Design review of the part built by this model. Coordinates are the model's own, in mm. Round coordinates to 2 decimals unless told otherwise and drop trailing zeros. Loops run counter-clockwise (first coordinate to the right, second up) from the corner with the lowest first, then second, coordinate; pieces in that order, holes last. Notation, with made-up numbers: M -20,-14 L 2,-14 A5 ccw 2,-7 Z; hole C 27.25,50.25 d3. An arc over 180 degrees is marked long. Answer as CSV lines item,"result". Start each with the question number.
from build123d import *

# Parameters (mm, degrees)
F0_R     = 24.5
F0_R_2   = 1.75
F0_R_3   = 1
F0_W     = 10
F0_H     = 24
F1_DEPTH = 6.35


with BuildPart() as f1:
    # F0 (on Top) → F1 (new body)
    with BuildSketch(Plane.XY):
        Circle(F0_R)
        with Locations((0, -18.5)):
            Circle(F0_R_2, mode=Mode.SUBTRACT)
        with Locations((-18.5, 0)):
            Circle(F0_R_2, mode=Mode.SUBTRACT)
        with Locations((-9, -9)):
            Circle(F0_R_3, mode=Mode.SUBTRACT)
        Rectangle(F0_W, F0_H, mode=Mode.SUBTRACT)
        with Locations((9, -9)):
            Circle(F0_R_3, mode=Mode.SUBTRACT)
        with Locations((18.5, 0)):
            Circle(F0_R_2, mode=Mode.SUBTRACT)
        with Locations((-9, 9)):
            Circle(F0_R_3, mode=Mode.SUBTRACT)
        with Locations((0, 18.5)):
            Circle(F0_R_2, mode=Mode.SUBTRACT)
        with Locations((9, 9)):
            Circle(F0_R_3, mode=Mode.SUBTRACT)
    extrude(amount=F1_DEPTH)


solid = f1.part
Item 1: Consider section A-A, the plane y = 0. Write out the cut boundary in (x, z).
Item 2: Insertion check: pin 1 Ø1.5 at (x, z) = (6.5, 2) entering from +Y; pin 2 Ø1.8 at (x, y) = (9, -9) entering from -Z; pin 3 Ø3 at (y, z) = (-5, 2.5) entering from -X; pin 4 Ø1.9 at (x, z) = (1.5, 3) entering from +Y. Each pin has a flat end and moves straight along its axis. Give the tip position at first contact, or say it passes through.
Item 3: Consider section B-B, the plane x = 9. Write out the cut boundary in (y, z).
Item 4: The part is to be moulded in two halves that separate along Z. For faces 1 (the face through (-9, 10, 3)), 2 (the face through (-6, 0, 6.35)), 3 (the face through (-6, 0, 0)), say which applies: +Z half, -Z half, draft (parallel to the pull), parting line (faces both ways), or undercut.
Item 5: Consider section D-D, the plane x = -18. Write out the cut boundary in (y, z), then the cut area to 3 significant figures.
Item 6: To check wall thickness, follow line 1 (Y direction, x = -9, z = 4); line 2 (Y direction, x = 0, z = 1.5); line 3 (X direction, y = -1.5, z = 3.25). State the ranges of each line that lie inside material, in increasing order.
Item 7: Consider section C-C, the plane z = 4. Count the separate pieces of the cut face and the enclosed holes in it, then the cut area to 3 significant figures.
Found:
1,outline,"M -24.5,0 L -20.25,0 L -20.25,6.35 L -24.5,6.35 Z; M -16.75,0 L -5,0 L -5,6.35 L -16.75,6.35 Z; M 5,0 L 16.75,0 L 16.75,6.35 L 5,6.35 Z; M 20.25,0 L 24.5,0 L 24.5,6.35 L 20.25,6.35 Z"
2,pin 1,"stops at y = 23.82"
2,pin 2,"passes through"
2,pin 3,"stops at x = -24.25"
2,pin 4,"stops at y = 24.49"
3,outline,"M -22.79,0 L -10,0 L -10,6.35 L -22.79,6.35 Z; M -8,0 L 8,0 L 8,6.35 L -8,6.35 Z; M 10,0 L 22.79,0 L 22.79,6.35 L 10,6.35 Z"
4,face 1,"draft"
4,face 2,"+Z half"
4,face 3,"-Z half"
5,outline,"M -16.62,0 L -1.68,0 L -1.68,6.35 L -16.62,6.35 Z; M 1.68,0 L 16.62,0 L 16.62,6.35 L 1.68,6.35 Z"
5,area,"190 mm^2"
6,line 1,"y = -22.79 to -10, -8 to 8, 10 to 22.79"
6,line 2,"y = -24.5 to -20.25, -16.75 to -12, 12 to 16.75, 20.25 to 24.5"
6,line 3,"x = -24.45 to -19.4, -17.6 to -5, 5 to 17.6, 19.4 to 24.45"
7,separate pieces,"1"
7,enclosed holes,"9"
7,area,"1,590 mm^2"
